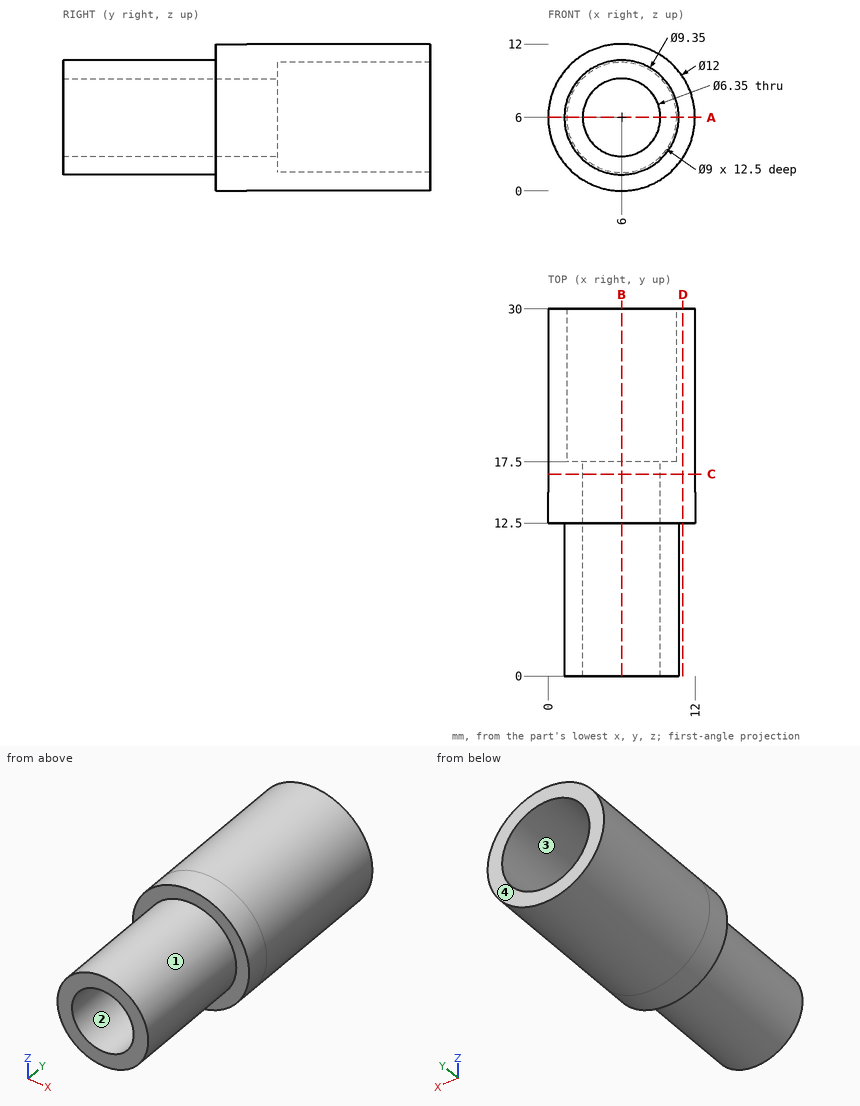
Source: three-view drawing plus pictorial views. Frame: mm from the lowest corner of the part. Round coordinates to 2 decimals unless told otherwise and drop trailing zeros. Write each loop counter-clockwise with the first axis right and the second up, starting at its lowest first coordinate (ties: lowest second). Pieces come first, ordered by that corner, then holes. Notation, with made-up numbers: (64.25, 46.25) -> (72.25, 46.25) arc R28 cw to (72.25, 74.25) -> close; hole circle Ø11 at (35, 76.5). An arc over 180 degrees is marked (long way). Return JSON: item names as keys, results as strings.
Q1. First-contact query: pin 1 Ø3 at (y, z) = (25.5, 8.5) entering from +X; pin 2 Ø1.5 at (y, z) = (3.5, 3.5) entering from -X; pin 3 Ø1 at (y, z) = (22, 8.5) entering from -X. Flat tips, straight axial feed; report the tip coordinate or a pass-through.
From the geometry:
{"pin 1": "x = 11.92", "pin 2": "x = 1.66", "pin 3": "x = 0.34"}
Q2. Section D-D on x = 11. Return the cut outline in (y, z), and give its area (3 significant figures).
From the geometry:
{"outline": "(12.5, 2.68) -> (30, 2.68) -> (30, 9.32) -> (12.5, 9.32) -> close", "area": "116 mm2"}
Q3. Ray query, line 1 (Z direction, x = 6, y = 25.5); line 2 (Y direction, x = 11.5, z = 7); line 3 (Z direction, x = 7.5, y = 27.25). Return the intervals inside material, ascending.
From the geometry:
{"line 1": "0 to 1.5, 10.5 to 12", "line 2": "12.5 to 30", "line 3": "0.19 to 1.76, 10.24 to 11.81"}
Q4. Section C-C on y = 16.5. Return the cut outline in (x, z) (3 decimals), and give its area (3 significant figures).
From the geometry:
{"outline": "circle Ø12 at (6, 6); hole circle Ø6.35 at (6, 6)", "area": "81.4 mm2"}
Q5. Mould query, pull axis X, two halves, no side actions, for the marked faces 1, 2, 3 and 4. Classes: +X half, -X half, draft (parallel to the pull), parting line (faces both ways), or undercut.
From the geometry:
{"face 1": "parting line", "face 2": "undercut", "face 3": "undercut", "face 4": "draft"}
Q6. Section B-B on x = 6. Return the cut outline in (y, z) (3 decimals).
From the geometry:
{"outline": "(0, 1.325) -> (12.5, 1.325) -> (12.5, 0) -> (30, 0) -> (30, 1.5) -> (17.5, 1.5) -> (17.5, 2.825) -> (0, 2.825) -> close; (0, 9.175) -> (17.5, 9.175) -> (17.5, 10.5) -> (30, 10.5) -> (30, 12) -> (12.5, 12) -> (12.5, 10.675) -> (0, 10.675) -> close"}
Q7. Section A-A on z = 6. Return the cut outline in (x, y) (3 decimals), and give its area (3 significant figures).
From the geometry:
{"outline": "(0, 12.5) -> (1.325, 12.5) -> (1.325, 0) -> (2.825, 0) -> (2.825, 17.5) -> (1.5, 17.5) -> (1.5, 30) -> (0, 30) -> close; (9.175, 0) -> (10.675, 0) -> (10.675, 12.5) -> (12, 12.5) -> (12, 30) -> (10.5, 30) -> (10.5, 17.5) -> (9.175, 17.5) -> close", "area": "103 mm2"}
